Can you work these out from the model? Positions are in its coordinate system, mm. Give positions to 0.01 mm unless a question says otherwise; leave off trailing zeros. Order: outer loops, then holes, each group sorted by start corner. A loop starts at its lowest first (then second) coordinate and runs counter-clockwise, first axis right, second up. Notation, with made-up numbers: M 4.25,37.25 L 12.25,37.25 A15 cw 12.25,49.25 Z; hole C -23,-36 d2. An arc over 180 degrees is marked long. Use one line per item in the form item = value. Start each with the question number.
1. I need wall thicknesses on L1, parallel to X at y = 6, z = 3; L2, parallel to X at y = -5, z = -7; L3, parallel to X at y = -1, z = 5.75. Which ranges of each line are inside material? Lowest first, please.
2. I want a section at C-C, the plane x = 539. List the corners of the cut face in (y, z) for me, and give its area (3 significant figures).
3. I want a section at B-B, the plane z = -0.25. List the corners of the cut face in (x, y) for me.
4. I want a section at A-A, the plane y = 0. List the corners of the cut face in (x, z) for me, and give its area (3 significant figures).
5. Will these pins go through, and if not, where does the flat tip stop? P1, Ø1.5, axis at y = 6, z = 7.5, coming from the +X side; P2, Ø1, axis at y = -6, z = -3.5, coming from the -X side; P3, Ø2, axis at x = 401, y = -2, coming from the +Z side.
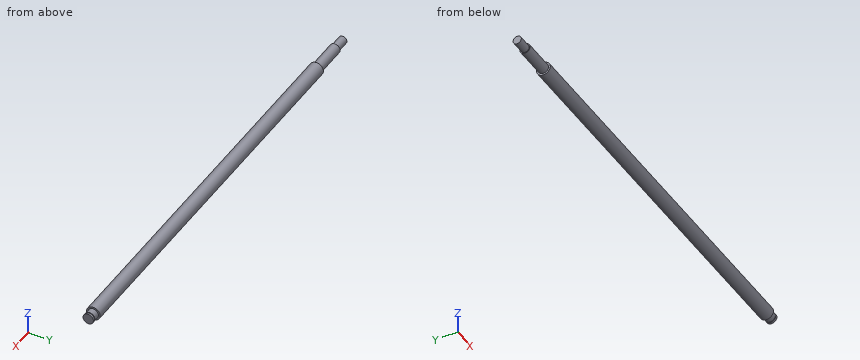
```python
from build123d import *

# Parameters (mm, degrees)
SKETCH_W      = 650
SKETCH_H      = 10
SKETCH001_W   = 67
SKETCH001_H   = 2.5
SKETCH002_W   = 20
SKETCH002_H   = 1.5
SKETCH003_W   = 13
SKETCH003_H   = 2.5
SKETCH003_W_2 = 1
SKETCH003_H_2 = 3.01


with BuildPart() as part:
    # Sketch → Revolution (revolve)
    with BuildSketch(Plane.XZ):
        with Locations((325, 5)):
            Rectangle(SKETCH_W, SKETCH_H)
    revolve(axis=Axis((0, 0, 0), (1, 0, 0)))

    # Sketch001 → Groove (revolve, cut)
    with BuildSketch(Plane.XZ):
        with Locations((33.5, 8.75)):
            Rectangle(SKETCH001_W, SKETCH001_H)
    revolve(axis=Axis((0, 0, 0), (1, 0, 0)), mode=Mode.SUBTRACT)

    # Sketch002 → Groove001 (revolve, cut)
    with BuildSketch(Plane.XZ):
        with Locations((10, 6.75)):
            Rectangle(SKETCH002_W, SKETCH002_H)
    revolve(axis=Axis((0, 0, 0), (1, 0, 0)), mode=Mode.SUBTRACT)

    # Sketch003 → Groove002 (revolve, cut)
    with BuildSketch(Plane.XZ):
        with Locations((643.5, 8.75)):
            Rectangle(SKETCH003_W, SKETCH003_H)
        with Locations((646.5, 5.995)):
            Rectangle(SKETCH003_W_2, SKETCH003_H_2)
    revolve(axis=Axis((0, 0, 0), (1, 0, 0)), mode=Mode.SUBTRACT)


solid = part.part
```
Check result:
q1.L1 = 20 to 646, 647 to 650
q1.L2 = 67 to 637
q1.L3 = 0 to 646, 647 to 650
q2.outline = C 0,0 d20
q2.area = 314 mm2
q3.outline = M 0,-5.99 L 20,-5.99 L 20,-7.5 L 67,-7.5 L 67,-10 L 637,-10 L 637,-7.5 L 646,-7.5 L 646,-4.48 L 647,-4.48 L 647,-7.5 L 650,-7.5 L 650,7.5 L 647,7.5 L 647,4.48 L 646,4.48 L 646,7.5 L 637,7.5 L 637,10 L 67,10 L 67,7.5 L 20,7.5 L 20,5.99 L 0,5.99 Z
q4.outline = M 0,-6 L 20,-6 L 20,-7.5 L 67,-7.5 L 67,-10 L 637,-10 L 637,-7.5 L 646,-7.5 L 646,-4.49 L 647,-4.49 L 647,-7.5 L 650,-7.5 L 650,7.5 L 647,7.5 L 647,4.49 L 646,4.49 L 646,7.5 L 637,7.5 L 637,10 L 67,10 L 67,7.5 L 20,7.5 L 20,6 L 0,6 Z
q4.area = 12,500 mm2
q5.P1 = 637
q5.P2 = 20
q5.P3 = 9.95
